Here's how the part is built. I have some questions about the finished solid (model axes, mm). A direction names the side the tool comes from. Coordinates: 2 decimals unless noted, no trailing zeros. Order: outer loops, then holes, each group sorted by start corner. A loop starts at its lowest first (then second) coordinate and runs counter-clockwise, first axis right, second up. Notation, with made-up numbers: (75.25, 37) -> (113.25, 37) arc R33 cw to (113.25, 68) -> close; hole circle Ø4 at (19, 12). An arc over 180 degrees is marked (long way). One line per item, written item: value. Start each with the question number.
Autodesk Inventor part; units mm, degrees
ref_plane "YZ Plane" through (0, 0, 0) normal (1, 0, 0) x (0, 1, 0)
ref_plane "XZ Plane" through (0, 0, 0) normal (0, 1, 0) x (-1, 0, 0)
ref_plane "XY Plane" through (0, 0, 0) normal (0, 0, 1) x (1, 0, 0)
sketch "Sketch1" plane through (0, 0, 0) normal (0, 0, 1) x (1, 0, 0)
  line L0 (0, 0) -> (124, 0)
  line L1 (124, 0) -> (124, 124)
  line L2 (124, 124) -> (0, 124)
  line L3 (0, 124) -> (0, 0)
  dimension "d0" = 124
  dimension "d1" = 124
extrude "Extrusion1" add sketch "Sketch1" along normal blind 10
sketch "Sketch2" plane through (0, 0, 10) normal (0, 0, 1) x (1, 0, 0)
  line L0 (0, 124) -> (0, 0)
  line L1 (0, 82) -> (-10, 82)
  line L2 (-10, 82) -> (-10, 42)
  line L3 (-10, 42) -> (0, 42)
  line L4 (0, 42) -> (0, 82)
  line L5 (0, 0) -> (124, 0)
  line L6 (42, 0) -> (82, 0)
  line L7 (82, 0) -> (82, -10)
  line L8 (82, -10) -> (42, -10)
  line L9 (42, -10) -> (42, 0)
  circle A0 centre (-5, 62) radius 2.5
  circle A1 centre (62, -5) radius 2.5
  point P0 (42, -5)
  point P1 (-10, 62)
  point P2 (-5, 82)
  point P3 (62, -10)
  point P4 (62, 0)
  point P5 (62, 0)
  point P6 (0, 62)
  dimension "d4" = 10
  dimension "d5" = 40
  dimension "d6" = 40
  dimension "d7" = 10
  dimension "d8" = 5
  dimension "d9" = 5
extrude "Extrusion2" add sketch "Sketch2" against normal blind 5
sketch "Sketch3" plane through (0, 0, 10) normal (0, 0, 1) x (1, 0, 0)
  line L0 (124, 124) -> (0, 124)
  line L1 (41, 124) -> (83, 124)
  line L2 (83, 124) -> (83, 112)
  line L3 (83, 112) -> (41, 112)
  line L4 (41, 112) -> (41, 124)
  point P0 (0, 0)
  point P1 (62, 112)
  point P2 (62, 124)
  dimension "d12" = 42
  dimension "d13" = 12
extrude "Extrusion3" cut sketch "Sketch3" against normal blind 6
sketch "Sketch4" plane through (0, 0, 4) normal (0, 0, 1) x (1, 0, 0)
  line L0 (41, 124) -> (83, 124) construction
  line L1 (41, 112) -> (41, 124) construction
  line L2 (83, 112) -> (41, 112) construction
  line L3 (83, 124) -> (83, 112) construction
  circle A0 centre (62, 119) radius 2.5
  point P0 (0, 0)
  point P1 (62, 124)
  dimension "d16" = 5
  dimension "d17" = 5
extrude "Extrusion4" cut sketch "Sketch4" against normal through all
sketch "Sketch5" plane through (0, 0, 10) normal (0, 0, 1) x (1, 0, 0)
  line L0 (124, 0) -> (124, 124)
  line L1 (124, 82) -> (134, 82)
  line L2 (134, 82) -> (134, 42)
  line L3 (134, 42) -> (124, 42)
  line L4 (124, 42) -> (124, 82)
  circle A0 centre (129, 62) radius 2.5
  point P0 (0, 0)
  point P1 (134, 62)
  point P2 (124, 62)
  point P3 (124, 62)
  point P4 (129, 82)
  dimension "d20" = 10
  dimension "d21" = 40
  dimension "d22" = 5
extrude "Extrusion5" add sketch "Sketch5" against normal blind 5
properties part number "TC006" material "ABS Plastic"
Q1. For faces 1 (the face through (-5, 82, 8)), 2 (the face through (62, 115, 4)), 3 (the face through (-5, 42, 8)), 4 (the face through (62, -2, 5)), 5 (the face through (82, -5, 8)), which set-ups out of +Z, -Z, +X, -X, +Y, -Y let a thin tool reach every point of the face, with its end or its side?
Q2. I need wall thicknesses on line 1 (Y direction, x = -5, z = 8.7); line 2 (X direction, y = 114, z = 8.25); line 3 (X direction, y = 65.5, z = 4.75). Which ranges of each line are inside material? Lowest first, please.
Q3. For P1, Ø2.5, axis at x = 131, z = 7.5, coming from the +Y side; P2, Ø2.5, axis at y = -7, z = 8.5, coming from the +X side; P3, Ø6, axis at x = 11.5, z = 1.5, coming from the -Y side; P4, Ø6, axis at x = 62, y = 119, coming from the -Z side, each with a flat end and sliding along its axis, tell me the tip position at first contact or that it passes through.
Q4. Imagine slicing it at A-A (x = 62). Write out the boundary of the cut face in (y, z), plus the area to 3 significant figures.
Q5. If we mould it in two halves opening along X, with no side actions, what happens to faces 6 (the face through (61.67, 121.48, 2.03)), 7 (the face through (-2.615, 62.751, 7.535)), 8 (the face through (-10, 62, 8)), 9 (the face through (61, 63, 0))? For each: +X half, -X half, draft (parallel to the pull), parting line (faces both ways), or undercut.
Q6. Imagine slicing it at D-D (x = -5). Write out the boundary of the cut face in (y, z).
Q7. Imagine slicing it at C-C (y = 119). Write out the boundary of the cut face in (x, z).
Q8. Imagine slicing it at B-B (z = 6.5). Write out the boundary of the cut face in (x, y), plus the area to 3 significant figures.
Completed:
1. face 1: +Z, -Z, -X, +Y
1. face 2: +Z, +Y
1. face 3: +Z, -Z, -X, -Y
1. face 4: -Z, +X, -X, -Y
1. face 5: +Z, -Z, +X, -Y
2. line 1: y = 42 to 59.5, 64.5 to 82
2. line 2: x = 0 to 41, 83 to 124
2. line 3: x = 0 to 124
3. P1: stops at y = 82
3. P2: stops at x = 82
3. P3: stops at y = 0
3. P4: stops at z = 0
4. outline: (-10, 5) -> (-7.5, 5) -> (-7.5, 10) -> (-10, 10) -> close; (-2.5, 5) -> (0, 5) -> (0, 0) -> (116.5, 0) -> (116.5, 4) -> (112, 4) -> (112, 10) -> (-2.5, 10) -> close; (121.5, 0) -> (124, 0) -> (124, 4) -> (121.5, 4) -> close
4. area: 1,170 mm2
5. face 6: undercut
5. face 7: undercut
5. face 8: -X half
5. face 9: draft
6. outline: (42, 5) -> (59.5, 5) -> (59.5, 10) -> (42, 10) -> close; (64.5, 5) -> (82, 5) -> (82, 10) -> (64.5, 10) -> close
7. outline: (0, 0) -> (59.5, 0) -> (59.5, 4) -> (41, 4) -> (41, 10) -> (0, 10) -> close; (64.5, 0) -> (124, 0) -> (124, 10) -> (83, 10) -> (83, 4) -> (64.5, 4) -> close
8. outline: (-10, 42) -> (0, 42) -> (0, 0) -> (42, 0) -> (42, -10) -> (82, -10) -> (82, 0) -> (124, 0) -> (124, 42) -> (134, 42) -> (134, 82) -> (124, 82) -> (124, 124) -> (83, 124) -> (83, 112) -> (41, 112) -> (41, 124) -> (0, 124) -> (0, 82) -> (-10, 82) -> close; hole circle Ø5 at (-5, 62); hole circle Ø5 at (62, -5); hole circle Ø5 at (129, 62)
8. area: 16,000 mm2
